Could you check a few things on this model? Use its own coordinates, in mm. A direction names the side the tool comes from. Give positions to 0.01 mm unless a question says otherwise; leave off trailing zeros. Loops run counter-clockwise (first coordinate to the right, second up) from the corner with the lowest first, then second, coordinate; pieces in that order, holes last. Notation, with made-up numbers: (53.5, 48.25) -> (75.5, 48.25) arc R16 ccw to (75.5, 61.25) -> close; hole circle Ø10 at (33, 18). An arc over 180 degrees is marked (long way). Write each question's results on one line, items separated by ' | '. Start each with the question number.
Q1. Will these pins go through, and if not, where does the flat tip stop? P1, Ø8, axis at y = 66.5, z = 88, coming from the -X side; P2, Ø8, axis at x = 89, z = 105.5, coming from the +Y side; P3, Ø1, axis at y = -159.5, z = 54.5, coming from the +X side.
Q2. If we section it at A-A, the plane z = 101.6: List the corners of the cut face in (x, y) for me.
Q3. Which directions (+Z, -Z, +X, -X, +Y, -Y) give clear straight access to the entire face, cutting with the end or side of a thin tool? Please do faces 1 (the face through (-102, -406.4, 101)), 2 (the face through (102, -406.4, 109)), 3 (the face through (-30.518, -644.322, 198.508)), 4 (the face through (164.25, -296.22, 14.49)).
Q4. If we section it at B-B, the plane y = -764.5: List the corners of the cut face in (x, z) for me, plus the area to 3 significant figures.
Q5. If I drill on line 1 along X through (y, z) = (0, 4); line 2 along Y through (x, z) = (0, 9); line 3 along X through (y, z) = (0, 5.5), over which ranges is the centre line in solid material (lowest first)?
Q6. We'd pull the mould along X, two halves only. Please class faces 5 (the face through (-122.955, -94.279, 195.907)), 6 (the face through (9.63, 317.354, 100.889)), 7 (the face through (-161.81, -299.81, 188.71)): released by +X, released by -X, zero draft, split by the parting line, or undercut.
from build123d import *

# Parameters (mm, degrees)
F0_R     = 154.94
F1_DEPTH = 203.2
F3_DEPTH = 508
F6_R     = 50.8


# Not quite as in the source:
# - a fillet or chamfer that OpenCascade refuses, or shapes differently, is made with other operations: its cross-section is extruded or revolved along the edge and cut away or added


with BuildPart() as f1:
    # F0 (on Top) → F1 (new body)
    with BuildSketch(Plane.XY):
        with BuildLine():
            Line((107.95, -406.4), (262.736611536, -178.2574625608))
            ThreePointArc((262.736611536, -178.2574625608), (0, 317.5), (-262.736611536, -178.2574625608))
            Line((-262.736611536, -178.2574625608), (-107.95, -406.4))
            Line((-107.95, -406.4), (0, -406.4))
            Line((0, -406.4), (107.95, -406.4))
        make_face()
        Circle(F0_R, mode=Mode.SUBTRACT)
    extrude(amount=F1_DEPTH)

    # F2 (on face) → F3 (join)
    with BuildSketch(Plane.XZ.offset(406.4)):
        with BuildLine():
            ThreePointArc((-6.5e-08, 0), (71.8420489456, 29.7579510085), (101.6, 101.6))
            ThreePointArc((101.6, 101.6), (71.8420489961, 173.442048941), (7.8e-08, 203.2))
            ThreePointArc((7.8e-08, 203.2), (-101.6, 101.6000000715), (-6.5e-08, 0))
        make_face()
    extrude(amount=F3_DEPTH)

    # F4 (on Right) → F5 (revolve, cut)
    with BuildSketch(Plane.YZ):
        with BuildLine():
            Line((0, 203.2), (-145.9118912221, 203.2))
            ThreePointArc((-145.9118912221, 203.2), (-177.8, 101.6), (-145.9118912221, 0))
            Line((-145.9118912221, 0), (0, 0))
            Line((0, 0), (0, 203.2))
        make_face()
    revolve(axis=Axis((0, 0, 101.6), (0, 0, -1)), mode=Mode.SUBTRACT)

    # F6
    f6_edges = [f1.edges().sort_by_distance(p)[0] for p in [
        (262.736612, -178.257463, 101.6),
        (-262.736612, -178.257463, 101.6),
        (0, 317.5, 0),
        (0, 317.5, 203.2),
        (-185.343306, -292.328731, 0),
        (-185.343306, -292.328731, 203.2),
        (185.343306, -292.328731, 0),
        (185.343306, -292.328731, 203.2),
    ]]
    fillet(f6_edges, radius=F6_R)

    # F7: chamfer of 25.4 on 1 edges, made by hand

    # F7_s1 → F7_t2 (revolve, cut)
    with BuildSketch(Plane.YZ):
        Polygon((-889, 0), (-914.4, 25.4), (-914.4, 0), align=None)
    revolve(axis=Axis((0, -914.4, 101.6), (0, 1, 0)), mode=Mode.SUBTRACT)


solid = f1.part
Final values:
1) P1: stops at x = -311.29 | P2: stops at y = 305.91 | P3: stops at x = 274.82
2) outline: (-262.74, -178.26) -> (-107.95, -406.4) -> (-101.6, -406.4) -> (-101.6, -889) -> (-76.2, -914.4) -> (76.2, -914.4) -> (101.6, -889) -> (101.6, -406.4) -> (107.95, -406.4) -> (262.74, -178.26) arc R317.5 ccw (long way) to start; hole circle Ø355.6 at (0, 0)
3) face 1: -X, -Y | face 2: +X, -Y | face 3: -Y | face 4: -Z, +X, -Y
4) outline: circle Ø203.2 at (0, 101.6) | area: 32,400 mm²
5) line 1: x = -286.46 to -154.94, 154.94 to 286.46 | line 2: y = -898 to -154.94, 154.94 to 295.57 | line 3: x = -289.69 to -154.94, 154.94 to 289.69
6) face 5: undercut | face 6: split by the parting line | face 7: released by -X
